from build123d import *

# Parameters (mm, degrees)
SKETCH1_W           = 36
SKETCH1_H           = 36
BOSS_EXTRUDE1_DEPTH = 3
SKETCH5_R           = 2
CUT_EXTRUDE3_DEPTH  = 10
SKETCH2_W           = 25
SKETCH2_H           = 25
CUT_EXTRUDE1_DEPTH  = 1
SKETCH4_W           = 11.5
SKETCH4_H           = 11.5
CUT_EXTRUDE4_DEPTH  = 3
SKETCH3_R           = 0.975
BOSS_EXTRUDE2_DEPTH = 5


with BuildPart() as part:
    # Sketch1 → Boss-Extrude1 (new body)
    with BuildSketch(Plane.XY):
        Rectangle(SKETCH1_W, SKETCH1_H)
    extrude(amount=BOSS_EXTRUDE1_DEPTH)

    # Sketch5 → Cut-Extrude3 (cut)
    with BuildSketch(Plane.XY.offset(3)):
        with Locations((-14, 14)):
            Circle(SKETCH5_R)
        with Locations((-14, -14)):
            Circle(SKETCH5_R)
        with Locations((14, -14)):
            Circle(SKETCH5_R)
        with Locations((14, 14)):
            Circle(SKETCH5_R)
    extrude(amount=-CUT_EXTRUDE3_DEPTH, mode=Mode.SUBTRACT)

    # Sketch2 → Cut-Extrude1 (cut)
    with BuildSketch(Plane.XY.offset(3)):
        Rectangle(SKETCH2_W, SKETCH2_H)
    extrude(amount=-CUT_EXTRUDE1_DEPTH, mode=Mode.SUBTRACT)

    # Sketch4 → Cut-Extrude4 (cut, through all)
    with BuildSketch(Plane.XY.offset(2)):
        with Locations((0, 2.75)):
            Rectangle(SKETCH4_W, SKETCH4_H)
    extrude(amount=-CUT_EXTRUDE4_DEPTH, mode=Mode.SUBTRACT)

    # Sketch3 → Boss-Extrude2 (add)
    with BuildSketch(Plane.XY.offset(2)):
        with Locations((10.1, 2.75)):
            Circle(SKETCH3_R)
        with Locations((10.1, -9.25)):
            Circle(SKETCH3_R)
        with Locations((-10.1, -9.25)):
            Circle(SKETCH3_R)
        with Locations((-10.1, 2.75)):
            Circle(SKETCH3_R)
    extrude(amount=BOSS_EXTRUDE2_DEPTH)


solid = part.part
Verification items for the finished model (mm, model axes). A direction names the side the tool comes from. Round coordinates to 2 decimals unless told otherwise and drop trailing zeros. Order: outer loops, then holes, each group sorted by start corner. A loop starts at its lowest first (then second) coordinate and runs counter-clockwise, first axis right, second up. Notation, with made-up numbers: (-27, 7.5) -> (20, 7.5) arc R5 cw to (20, 12.5) -> close; hole circle Ø4 at (2.5, 67.25). An arc over 180 degrees is marked (long way). Put each result on its own line as item: value.
1) Depth check by flat-ended pin: pin 1 (3 mm diameter, centred on y = 8, z = 5, fed in from -X); pin 2 (1.5 mm diameter, centred on x = -11.5, z = 4.5, fed in from +Y). Enter the tip coordinate at first touch or a pass-through.
Final values:
pin 1: passes through
pin 2: stops at y = 3.48
2) Section check B-B (x = 14). Record the cut outline in (y, z).
Final values:
outline: (-18, 0) -> (-16, 0) -> (-16, 3) -> (-18, 3) -> close; (-12, 0) -> (12, 0) -> (12, 3) -> (-12, 3) -> close; (16, 0) -> (18, 0) -> (18, 3) -> (16, 3) -> close
3) Material ranges on line 1 (Y direction, x = -14, z = 2.25); line 2 (Z direction, x = 9, y = -8); line 3 (X direction, y = -8, z = 2.5), recorded low to high.
Final values:
line 1: y = -18 to -16, -12 to 12, 16 to 18
line 2: z = 0 to 2
line 3: x = -18 to -12.5, 12.5 to 18
4) Section check A-A (y = 2.75). Record the cut outline in (x, z) (3 decimals), then the cut area to 3 significant figures.
Final values:
outline: (-18, 0) -> (-5.75, 0) -> (-5.75, 2) -> (-9.125, 2) -> (-9.125, 7) -> (-11.075, 7) -> (-11.075, 2) -> (-12.5, 2) -> (-12.5, 3) -> (-18, 3) -> close; (5.75, 0) -> (18, 0) -> (18, 3) -> (12.5, 3) -> (12.5, 2) -> (11.075, 2) -> (11.075, 7) -> (9.125, 7) -> (9.125, 2) -> (5.75, 2) -> close
area: 79.5 mm^2
5) Set-up check for faces 3 (the flat face through (0, -3, 1)), 4 (the cylindrical face through (9.326, -9.843, 4.465)), 5 (the flat face through (0, -4, 0)): record each of +Z, -Z, +X, -X, +Y, -Y from which the full face is reachable in a straight line by a thin tool's end or side.
Final values:
face 3: +Z, -Z
face 4: +Z
face 5: -Z, +X, -X, +Y, -Y
6) Section check D-D (x = -7). Record the cut outline in (y, z), then the cut area to 3 significant figures.
Final values:
outline: (-18, 0) -> (18, 0) -> (18, 3) -> (12.5, 3) -> (12.5, 2) -> (-12.5, 2) -> (-12.5, 3) -> (-18, 3) -> close
area: 83.0 mm^2
7) Mould release check, pull along Y, two halves, no side actions. Record for faces 1 (the flat face through (-0.2, -12.5, 2.5)), 2 (the flat face through (-18, 0, 1)): +Y half, -Y half, draft (parallel to the pull), parting line (faces both ways), or undercut.
Final values:
face 1: undercut
face 2: draft
